Part model, mm, in its own coordinate system. Coordinates: 2 decimals unless noted, no trailing zeros. Use a Markdown table: item, result. Add a question column.
1) Wall check: probe 1 along X at (y, z) = (2, -17); probe 2 along Z at (x, y) = (-37.5, 1.1); probe 3 along Z at (x, y) = (-38, 0.2). Give the ranges that are in metal, low to high. Write a range as from..to.
2) Pull direction Z, two halves, no side cores. Call faces 1 (the flat face through (42.5, 1, 0)), 2 (the cylindrical face through (37.292, 1.521, 15.414)), 3 (the flat face through (-1, 1, -22)): released by +Z, released by -Z, zero draft, split by the parting line, or undercut.
3) Pin check, flat tip, straight feed: pin 1 Ø3 at (x, z) = (-37.5, -17) entering from -Y. Stop position of the tip, or through.
from build123d import *

# Parameters (mm, degrees)
SKETCH_1_W          = 85
SKETCH_1_H          = 44
EXTRUDE_1_DEPTH     = 3
SKETCH_2_R          = 1.6
CUT_EXTRUDE_1_DEPTH = 4
FILLET_1_R          = 5


with BuildPart() as part:
    # 草图1 → 凸台-拉伸1 (new body)
    with BuildSketch(Plane(origin=(0, 0, 0), x_dir=(1, 0, 0), z_dir=(0, 1, 0))):
        Rectangle(SKETCH_1_W, SKETCH_1_H)
    extrude(amount=EXTRUDE_1_DEPTH)

    # 草图2 → 切除-拉伸1 (cut, through all)
    with BuildSketch(Plane(origin=(0, 3, 0), x_dir=(1, 0, 0), z_dir=(0, 1, 0))):
        with Locations((-37.5, 17)):
            Circle(SKETCH_2_R)
        with Locations((-37.5, -17)):
            Circle(SKETCH_2_R)
        with Locations((37.5, 17)):
            Circle(SKETCH_2_R)
        with Locations((37.5, -17)):
            Circle(SKETCH_2_R)
    extrude(amount=-CUT_EXTRUDE_1_DEPTH, mode=Mode.SUBTRACT)

    # 圆角1
    fillet_1_edges = [part.edges().sort_by_distance(p)[0] for p in [
        (-42.5, 1.5, -22),
        (42.5, 1.5, -22),
        (42.5, 1.5, 22),
        (-42.5, 1.5, 22),
    ]]
    fillet(fillet_1_edges, radius=FILLET_1_R)


solid = part.part
Entries:
| question | item | result |
|---|---|---|
| 1 | probe 1 | -42.5..-39.1, -35.9..35.9, 39.1..42.5 |
| 1 | probe 2 | -22..-18.6, -15.4..15.4, 18.6..22 |
| 1 | probe 3 | -21.97..-18.52, -15.48..15.48, 18.52..21.97 |
| 2 | face 1 | zero draft |
| 2 | face 2 | undercut |
| 2 | face 3 | released by -Z |
| 3 | pin 1 | through |
